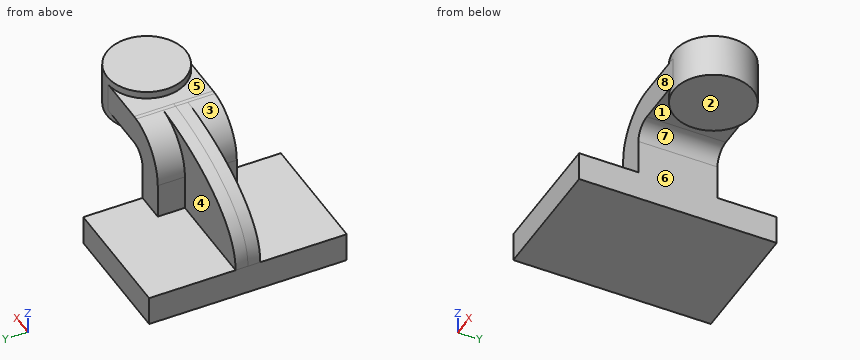
```python
from build123d import *

# Parameters (mm, degrees)
F1_DEPTH = 63.5
F2_DEPTH = 25.4
F0_W     = 25.3816735625
F0_H     = 19.05
F3_DEPTH = 25.4
F5_DEPTH = 7.9375


with BuildPart() as f1:
    # F0 (on Front) → F1 (new body, symmetric)
    with BuildSketch(Plane.XZ):
        Polygon((41.275, -9.525), (41.275, 9.525), (22.225, 9.525), (-41.275, 9.525), (-41.275, -9.525), align=None)
    extrude(amount=F1_DEPTH, both=True)

    # F0 (on Front) → F2 (join, symmetric)
    with BuildSketch(Plane.XZ):
        with BuildLine():
            Line((22.225, 9.525), (41.275, 9.525))
            Line((41.275, 9.525), (41.275, 32.3611232806))
            ThreePointArc((41.275, 32.3611232806), (44.3545017732, 39.7956982268), (51.7890767194, 42.8752))
            Line((51.7890767194, 42.8752), (60.325, 42.8752))
            Line((60.325, 42.8752), (60.325, 61.9252))
            Line((60.325, 61.9252), (51.7890767194, 61.9252))
            add(Edge.make_bspline(
                [(49.378379009, 61.8267501842), (50.188059931, 61.8657540614), (50.9918272392, 61.8985579588), (51.7890767194, 61.9252)],
                knots=[104.6145771786, 104.6145771786, 104.6145771786, 104.6145771786, 106.8021691525, 106.8021691525, 106.8021691525, 106.8021691525], degree=3))
            ThreePointArc((49.378379009, 61.8267501842), (30.0485076798, 52.3956507296), (22.225, 32.3611232806))
            Line((22.225, 32.3611232806), (22.225, 9.525))
        make_face()
    extrude(amount=F2_DEPTH, both=True)

    # F0 (on Front) → F3 (join, symmetric)
    with BuildSketch(Plane.XZ):
        with Locations((73.0158367813, 52.4002)):
            Rectangle(F0_W, F0_H)
    extrude(amount=F3_DEPTH, both=True)

    # F0 (on Front) → F4 (revolve)
    with BuildSketch(Plane.XZ):
        Polygon((85.7066735625, 61.9252), (85.7066735625, 42.8752), (85.7066735625, 38.1), (111.125, 38.1), (111.125, 66.675), (85.7066735625, 66.675), align=None)
    revolve(axis=Axis((85.7066735625, 0, 52.3875), (0, 0, -1)))

    # F0 (on Front) → F5 (join, symmetric)
    with BuildSketch(Plane.XZ):
        with BuildLine():
            Line((-41.275, 9.525), (22.225, 9.525))
            Line((22.225, 9.525), (22.225, 32.3611232806))
            ThreePointArc((22.225, 32.3611232806), (30.0485076798, 52.3956507296), (49.378379009, 61.8267501842))
            add(Edge.make_bspline(
                [(-41.275, 9.525), (-41.5863992268, 43.9173953964), (10.6579831052, 59.9615147216), (49.378379009, 61.8267501842)],
                knots=[0, 0, 0, 0, 104.6145771786, 104.6145771786, 104.6145771786, 104.6145771786], degree=3))
        make_face()
    extrude(amount=F5_DEPTH, both=True)


solid = f1.part
```
CAD build for the part. Positions are in the model's coordinates, mm. Face numbers are marked on the shaded views. A direction names the side the tool comes from. Round coordinates to 2 decimals unless told otherwise and drop trailing zeros. Write each loop counter-clockwise with the first axis right and the second up, starting at its lowest first coordinate (ties: lowest second). Pieces come first, ordered by that corner, then holes. Notation, with made-up numbers: (85, 44.5) -> (130, 44.5) arc R27 cw to (130, 71.5) -> close; hole circle Ø10 at (32.25, 24). An arc over 180 degrees is marked (long way). Answer in a Markdown table with one row per item. Add a question column.
Item 1: Saw through at A-A, the plane x = 100.5. Write the cut outline in (y, z) (3 decimals).
Item 2: Saw through at B-B, the plane y = 36.5. Write the cut outline in (x, z) (3 decimals), then the cut area to 3 significant figures.
Item 3: Saw through at C-C, the plane x = 81.5. Write the cut outline in (y, z) (3 decimals).
Item 4: Mould opens along X. For the marked faces 1, 2 and 3 say: pulls with the +X half, pulls with the -X half, needs draft (parallel to the pull), parting line crosses it, or undercut.
Item 5: Drop flat-ended pins along their axis: pin 1 Ø16.5 at (x, y) = (67, 6.5) entering from -Z; pin 2 Ø15.5 at (x, z) = (-5.5, 26) entering from -Y; pin 3 Ø5 at (x, z) = (60, 44) entering from -Y. Give the stop position or say it passes through.
Item 6: Which spindle directions (+Z, -Z, +X, -X, +Y, -Y) get a long thin tool onto all of the face, cutting with end or side? Do the marked faces 4, 5, 6, 7 and 8. Say none if no direction does.
Item 7: Drill centre lines: line 1 (Z direction, x = -33.5, y = -48) (3 decimals); line 2 (X direction, y = 25, z = 4) (3 decimals); line 3 (Z direction, x = 98, y = -22) (3 decimals). Where is each one in solid material? Low to high. Write a range as from..to.
Findings below:
| question | item | result |
|---|---|---|
| 1 | outline | (-20.67, 38.1) -> (20.67, 38.1) -> (20.67, 66.675) -> (-20.67, 66.675) -> close |
| 2 | outline | (-41.275, -9.525) -> (41.275, -9.525) -> (41.275, 9.525) -> (-41.275, 9.525) -> close |
| 2 | area | 1,570 mm^2 |
| 3 | outline | (-25.4, 42.875) -> (-25.068, 42.875) -> (-25.068, 38.1) -> (25.068, 38.1) -> (25.068, 42.875) -> (25.4, 42.875) -> (25.4, 61.925) -> (25.068, 61.925) -> (25.068, 66.675) -> (-25.068, 66.675) -> (-25.068, 61.925) -> (-25.4, 61.925) -> close |
| 4 | face 1 | undercut |
| 4 | face 2 | needs draft |
| 4 | face 3 | pulls with the -X half |
| 5 | pin 1 | stops at z = 38.1 |
| 5 | pin 2 | stops at y = -7.94 |
| 5 | pin 3 | stops at y = -25.4 |
| 6 | face 4 | +Z, -X, +Y |
| 6 | face 5 | +Z, -X |
| 6 | face 6 | -Z, +X, +Y, -Y |
| 6 | face 7 | -Z, +Y, -Y |
| 6 | face 8 | +Z, +X, -X, -Y |
| 7 | line 1 | z = -9.525..9.525 |
| 7 | line 2 | x = -41.275..41.275 |
| 7 | line 3 | z = 38.1..66.675 |
